Check sheet for the modelled part. Datum: model origin and axes. Units: mm. Round coordinates to 2 decimals unless told otherwise and drop trailing zeros. Write each loop counter-clockwise with the first axis right and the second up, starting at its lowest first coordinate (ties: lowest second). Pieces come first, ordered by that corner, then holes.
Item 1: Go/stop test with flat-tipped pins: pin 1 Ø3.5 at (x, y) = (95.25, 95.25) entering from -Z; pin 2 Ø4 at (x, y) = (95.25, 6.35) entering from -Z. Record where each tip stops, or that it passes through.
Item 2: Material ranges on line 1 (Y direction, x = 6.35, z = 2.75); line 2 (X direction, y = 96, z = 1.15); line 3 (Y direction, x = 5, z = 4.3), recorded low to high.
Item 3: Release check for a two-part mould opening along Y. For faces 1 (the cylindrical face through (1.449, 1.528, 2.576)), 2 (the cylindrical face through (5.951, 93.452, 2.576)), 3 (the cylindrical face through (100.072, 100.151, 2.576)) record: +Y half, -Y half, draft (parallel to the pull), parting line (faces both ways), or undercut.
Item 4: Cross-section at A-A on x = 6.35. Enter the section's corners in (y, z).
from build123d import *

# Parameters (mm, degrees)
F0_W     = 101.6
F0_H     = 101.6
F1_DEPTH = 5.08
F2_R     = 1.8415
F3_DEPTH = 5.081
F4_R     = 5.08


with BuildPart() as f1:
    # F0 (on Top) → F1 (new body)
    with BuildSketch(Plane.XY):
        with Locations((50.8, 50.8)):
            Rectangle(F0_W, F0_H)
    extrude(amount=F1_DEPTH)

    # F2 (on face) → F3 (cut, through all)
    with BuildSketch(Plane.XY.offset(5.08)):
        with Locations((6.35, 95.25)):
            Circle(F2_R)
        with Locations((95.25, 95.25)):
            Circle(F2_R)
        with Locations((95.25, 6.35)):
            Circle(F2_R)
        with Locations((6.35, 6.35)):
            Circle(F2_R)
    extrude(amount=-F3_DEPTH, mode=Mode.SUBTRACT)

    # F4
    f4_edges = [f1.edges().sort_by_distance(p)[0] for p in [
        (0, 0, 2.54),
        (101.6, 0, 2.54),
        (101.6, 101.6, 2.54),
        (0, 101.6, 2.54),
    ]]
    fillet(f4_edges, radius=F4_R)


solid = f1.part
Response values:
1. pin 1: passes through
1. pin 2: stops at z = 0
2. line 1: y = 0 to 4.51, 8.19 to 93.41, 97.09 to 101.6
2. line 2: x = 0 to 4.67, 8.03 to 93.57, 96.93 to 101.6
2. line 3: y = 0 to 5.1, 7.6 to 94, 96.5 to 101.6
3. face 1: -Y half
3. face 2: undercut
3. face 3: +Y half
4. outline: (0, 0) - (4.51, 0) - (4.51, 5.08) - (0, 5.08) - close; (8.19, 0) - (93.41, 0) - (93.41, 5.08) - (8.19, 5.08) - close; (97.09, 0) - (101.6, 0) - (101.6, 5.08) - (97.09, 5.08) - close
